Geometry check sheet. Reference: the model listing, model coordinates, mm. Coordinates: 2 decimals unless noted, no trailing zeros. Loops run counter-clockwise (first coordinate to the right, second up) from the corner with the lowest first, then second, coordinate; pieces in that order, holes last. Notation, with made-up numbers: (-27, 5) - (32, 5) arc R18 cw to (32, 14) - close; hole circle Ø7 at (-33.75, -35). An arc over 180 degrees is marked (long way). One line per item, written item: value.
Autodesk Inventor part; units mm, degrees
ref_plane "YZ Plane" through (0, 0, 0) normal (1, 0, 0) x (0, 1, 0)
ref_plane "XZ Plane" through (0, 0, 0) normal (0, 1, 0) x (-1, 0, 0)
ref_plane "XY Plane" through (0, 0, 0) normal (0, 0, 1) x (1, 0, 0)
sketch "スケッチ1" plane through (0, 0, 0) normal (0, 0, 1) x (1, 0, 0)
  circle A0 centre (0, 0) radius 7.5
  circle A1 centre (0, 0) radius 5 construction
  circle A2 centre (0, 5) radius 0.8
  circle A3 centre (-3.5355, 3.5355) radius 0.8
  circle A4 centre (-5, 0) radius 0.8
  circle A5 centre (-3.5355, -3.5355) radius 0.8
  circle A6 centre (0, -5) radius 0.8
  circle A7 centre (3.5355, -3.5355) radius 0.8
  circle A8 centre (5, 0) radius 0.8
  circle A9 centre (3.5355, 3.5355) radius 0.8
  circle A10 centre (0, 0) radius 1.3
  dimension "d1" = 10
  dimension "d0" = 15
  dimension "d2" = 1.6
  dimension "d5" = 360
  dimension "d7" = 2.6
extrude "押し出し1" add sketch "スケッチ1" along normal blind 3
properties part number "dentatu"
(1) Release check for a two-part mould opening along Y. For faces 1 (the face through (-7.493, -0.33, 1.479)), 2 (the face through (0, -2, 0)), 3 (the face through (3.431, 2.742, 1.479)), 4 (the face through (3.43, -4.33, 1.48)) record: pulls with the +Y half, pulls with the -Y half, needs draft (parallel to the pull), parting line crosses it, or undercut.
Reply:
face 1: parting line crosses it
face 2: needs draft
face 3: undercut
face 4: undercut
(2) Cross-section at A-A on y = 0. Record the cut outline in (x, z).
Reply:
outline: (-7.5, 0) - (-5.8, 0) - (-5.8, 3) - (-7.5, 3) - close; (-4.2, 0) - (-1.3, 0) - (-1.3, 3) - (-4.2, 3) - close; (1.3, 0) - (4.2, 0) - (4.2, 3) - (1.3, 3) - close; (5.8, 0) - (7.5, 0) - (7.5, 3) - (5.8, 3) - close
(3) Cross-section at C-C on z = 1.45. State how many separate pieces and enclosed holes the cut face has, and give its area (3 significant figures).
Reply:
separate pieces: 1
enclosed holes: 9
area: 155 mm2
(4) Go/stop test with flat-tipped pins: pin 1 Ø2 at (x, y) = (2.5, 0.5) entering from -Z; pin 2 Ø1.3 at (x, y) = (0, -5) entering from +Z; pin 3 Ø1 at (y, z) = (-2.5, 1) entering from -X. Record where each tip stops, or that it passes through.
Reply:
pin 1: z = 0
pin 2: through
pin 3: x = -7.23
(5) Cross-section at D-D on x = 5. Record the cut outline in (y, z).
Reply:
outline: (-5.59, 0) - (-0.8, 0) - (-0.8, 3) - (-5.59, 3) - close; (0.8, 0) - (5.59, 0) - (5.59, 3) - (0.8, 3) - close
(6) Material ranges on probe 1 along Y at (x, z) = (0, 2.3); probe 2 along X at (y, z) = (-0.5, 0.15); probe 3 along X at (y, z) = (4, 2.5), recorded low to high. Write a range as from..to.
Reply:
probe 1: -7.5..-5.8, -4.2..-1.3, 1.3..4.2, 5.8..7.5
probe 2: -7.48..-5.62, -4.38..-1.2, 1.2..4.38, 5.62..7.48
probe 3: -6.34..-4.19, -2.88..2.88, 4.19..6.34
